from build123d import *

# Parameters (mm, degrees)
F1_DEPTH = 24.5
F2_W     = 24
F2_H     = 5.8
F3_DEPTH = 2
F4_W     = 24
F4_H     = 11
F4_W_2   = 4.5
F4_H_2   = 2
F5_DEPTH = 2
F6_DEPTH = 1


# Not quite as in the source:
# - a feature of the source that left no trace in its solid (it failed there, or was rolled back) is left out


with BuildPart() as f1:
    # F0 (on Front) → F1 (new body)
    with BuildSketch(Plane.XZ):
        Polygon((-6.75, 2.2), (-6.75, 4.5), (-4.85, 4.5), (-3.2, 4.5), (3.2, 4.5), (4.85, 4.5), (6.75, 4.5), (6.75, 2.2), (4.85, 2.2), (4.85, 0.7), (12.25, 0.7), (12.25, 6.5), (-11.75, 6.5), (-11.75, 0.7), (-4.85, 0.7), (-4.85, 2.2), align=None)
    extrude(amount=F1_DEPTH)

    # F2 (on face) → F3 (join)
    with BuildSketch(Plane.XZ.offset(24.5)):
        with Locations((0.25, 3.6)):
            Rectangle(F2_W, F2_H)
    extrude(amount=F3_DEPTH)

    # F4 (on face) → F5 (join)
    with BuildSketch(Plane.XY.offset(6.5)):
        with Locations((0.25, 5.5)):
            Rectangle(F4_W, F4_H)
        with Locations((0, 7.5)):
            Rectangle(F4_W_2, F4_H_2, mode=Mode.SUBTRACT)
    extrude(amount=-F5_DEPTH)

    # F4 (on face) → F6 (join)
    with BuildSketch(Plane.XY.offset(6.5)):
        with Locations((0, 7.5)):
            Rectangle(F4_W_2, F4_H_2)
    extrude(amount=-F6_DEPTH)


solid = f1.part
Model file for the job. Use its own axes, mm. A direction names the side the tool comes from. Give positions to 0.01 mm unless a question says otherwise; leave off trailing zeros. Loops run counter-clockwise (first coordinate to the right, second up) from the corner with the lowest first, then second, coordinate; pieces in that order, holes last. Notation, with made-up numbers: (36, 84.5) -> (72, 84.5) arc R18 ccw to (72, 101.5) -> close; hole circle Ø1 at (-23, -37.75). An arc over 180 degrees is marked (long way). Use a Markdown table: item, result. Add a question column.
(1) Tool access for faces 5 (the flat face through (-9, 0, 3)), 6 (the flat face through (0, -3, 4.5)), 7 (the flat face through (0, 6.5, 5)), 8 (the flat face through (-4.85, -12, 1)): list every direction of +Z, -Z, +X, -X, +Y, -Y with a clear straight run to the whole face (end or side of a thin tool).
(2) Wall check: line 1 along X through (y, z) = (-3.5, 0.9); line 2 along Z through (x, y) = (-5.75, -1); line 3 along Z through (x, y) = (-3.5, -10.5). Give the ranges that are in metal, low to high.
(3) Slice it at D-D on x = 9.5. List the corners of the cut face in (y, z), and give its area (3 significant figures).
(4) Slice it at C-C on y = -19. List the corners of the cut face in (x, z).
(5) Slice it at A-A on x = -0.25. List the corners of the cut face in (y, z).
(6) Slice it at B-B on z = 1.65. List the corners of the cut face in (x, y), and give its area (3 significant figures).
(7) Mould opens along Z. For faces 1 (the flat face through (2.25, 7, 5)), 2 (the flat face through (-6, -12, 2.2)), 3 (the flat face through (0, -24.5, 3)), 4 (the flat face through (0, -7, 6.5)) say: +Z half, -Z half, draft (parallel to the pull), parting line (faces both ways), or undercut.
(8) Drop flat-ended pins along their axis: pin 1 Ø1.9 at (x, z) = (8.5, 2) entering from +Y; pin 2 Ø0.6 at (x, y) = (0.5, 7.5) entering from -Z. Give the stop position or say it passes through.
Filled sheet:
| question | item | result |
|---|---|---|
| 1 | face 5 | -Z, +X, -X, +Y |
| 1 | face 6 | +Y |
| 1 | face 7 | -Z |
| 1 | face 8 | -Z, +Y |
| 2 | line 1 | -11.75 to -4.85, 4.85 to 12.25 |
| 2 | line 2 | 0.7 to 2.2, 4.5 to 6.5 |
| 2 | line 3 | 4.5 to 6.5 |
| 3 | outline | (-26.5, 0.7) -> (0, 0.7) -> (0, 4.5) -> (11, 4.5) -> (11, 6.5) -> (-26.5, 6.5) -> close |
| 3 | area | 176 mm2 |
| 4 | outline | (-11.75, 0.7) -> (-4.85, 0.7) -> (-4.85, 2.2) -> (-6.75, 2.2) -> (-6.75, 4.5) -> (6.75, 4.5) -> (6.75, 2.2) -> (4.85, 2.2) -> (4.85, 0.7) -> (12.25, 0.7) -> (12.25, 6.5) -> (-11.75, 6.5) -> close |
| 5 | outline | (-26.5, 0.7) -> (-24.5, 0.7) -> (-24.5, 4.5) -> (6.5, 4.5) -> (6.5, 5.5) -> (8.5, 5.5) -> (8.5, 4.5) -> (11, 4.5) -> (11, 6.5) -> (-26.5, 6.5) -> close |
| 6 | outline | (-11.75, -26.5) -> (12.25, -26.5) -> (12.25, 0) -> (4.85, 0) -> (4.85, -24.5) -> (-4.85, -24.5) -> (-4.85, 0) -> (-11.75, 0) -> close |
| 6 | area | 398 mm2 |
| 7 | face 1 | draft |
| 7 | face 2 | undercut |
| 7 | face 3 | undercut |
| 7 | face 4 | +Z half |
| 8 | pin 1 | y = 0 |
| 8 | pin 2 | z = 5.5 |
